Can you work these out from the model? Positions are in its coordinate system, mm. Give positions to 0.01 mm unless a question says otherwise; leave off trailing zeros. Loops run counter-clockwise (first coordinate to the right, second up) from the corner with the lowest first, then second, coordinate; pieces in that order, holes last. Notation, with made-up numbers: M -19,56 L 3,56 A32 ccw 3,94 Z; hole C 15,33.25 d7. An arc over 180 degrees is marked long. Put each result on its own line as item: value. Start each with the question number.
1) Imagine slicing it at A-A (y = 14.25). Write out the boundary of the cut face in (x, z), then the cut area to 3 significant figures.
2) Please list where these lines run through material, in increasing order: line 1 along Y through (x, z) = (-0.7, -0.2); line 2 along Z through (x, y) = (0.1, 5.25); line 3 along Y through (x, z) = (-0.1, -1.7). Write a range as from..to.
3) For P1, Ø1.1, axis at x = 1, y = 17.5, coming from the +Z side; P2, Ø2, axis at x = 1, y = 5.5, coming from the -Z side; P3, Ø0.5, axis at y = 17.5, z = 1, coming from the -X side; P4, Ø1.3, axis at x = 0.5, z = 1, coming from the -Y side, each with a flat end and sliding along its axis, tell me the tip position at first contact or that it passes through.
4) If we mould it in two halves opening along X, with no side actions, what happens to faces 1 (the flat face through (0.375, 17.4, 1.1)), 2 (the cylindrical face through (1.5, 8.23, 0.07)), 3 (the flat face through (0, 0, 0))? For each: +X half, -X half, draft (parallel to the pull), parting line (faces both ways), or undercut.
from build123d import *

# Parameters (mm, degrees)
CHAMFER1_SIZE      = 0.5
CUT_EXTRUDE3_DEPTH = 1


with BuildPart() as part:
    # Sketch1 → Revolve1 (revolve)
    with BuildSketch(Plane.XY):
        with BuildLine():
            Line((0, 0), (-1.5, 0))
            Line((-1.5, 0), (-1.5, 15.75))
            ThreePointArc((-1.5, 15.75), (-1.573223305, 15.926776695), (-1.75, 16))
            Line((-1.75, 16), (-2.132389685, 16))
            ThreePointArc((-2.132389685, 16), (-2.321151019, 16.086081853), (-2.379920949, 16.285046729))
            ThreePointArc((-2.379920949, 16.285046729), (-1.555396609, 17.649656197), (0, 18))
            Line((0, 18), (0, 0))
        make_face()
    revolve(axis=Axis((0, 0, 0), (0, 1, 0)))

    # Chamfer1
    chamfer1_edges = [part.edges().sort_by_distance(p)[0] for p in [
        (1.5, 0, 0),
    ]]
    chamfer(chamfer1_edges, length=CHAMFER1_SIZE)

    # Sketch9 → Cut-Extrude3 (cut)
    with BuildSketch(Plane(origin=(0, 18.033333333, 0), x_dir=(1, 0, 0), z_dir=(0, 1, 0))):
        with BuildLine():
            Line((-0.375, 1.875), (0.375, 1.875))
            Line((0.375, 1.875), (0.375, 0.625))
            ThreePointArc((0.375, 0.625), (0.448223305, 0.448223305), (0.625, 0.375))
            Line((0.625, 0.375), (1.875, 0.375))
            Line((1.875, 0.375), (1.875, -0.375))
            Line((1.875, -0.375), (0.625, -0.375))
            ThreePointArc((0.625, -0.375), (0.448223305, -0.448223305), (0.375, -0.625))
            Line((0.375, -0.625), (0.375, -1.875))
            Line((0.375, -1.875), (-0.375, -1.875))
            Line((-0.375, -1.875), (-0.375, -0.625))
            ThreePointArc((-0.375, -0.625), (-0.448223305, -0.448223305), (-0.625, -0.375))
            Line((-0.625, -0.375), (-1.875, -0.375))
            Line((-1.875, -0.375), (-1.875, 0.375))
            Line((-1.875, 0.375), (-0.625, 0.375))
            ThreePointArc((-0.625, 0.375), (-0.448223305, 0.448223305), (-0.375, 0.625))
            Line((-0.375, 0.625), (-0.375, 1.875))
        make_face()
    extrude(amount=-CUT_EXTRUDE3_DEPTH, mode=Mode.SUBTRACT)


solid = part.part
Recorded:
1. outline: C 0,0 d3
1. area: 7.07 mm²
2. line 1: 0..17.03
2. line 2: -1.5..1.5
2. line 3: 16..17.03
3. P1: z = 2
3. P2: z = -1.5
3. P3: x = -1.74
3. P4: y = 0
4. face 1: undercut
4. face 2: parting line
4. face 3: draft
